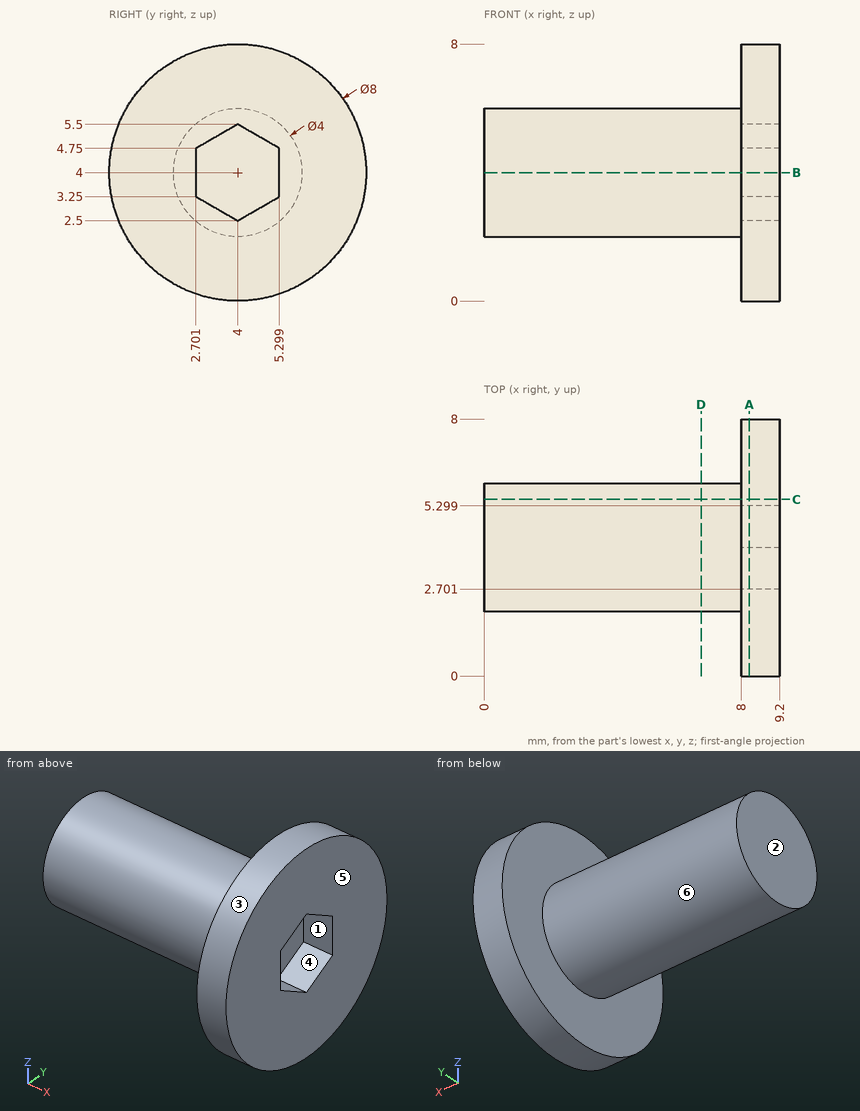
Could you check a few things on this drawing? It's one solid part, dimensions in mm from its lowest x, y, z. A direction names the side the tool comes from. Round coordinates to 2 decimals unless told otherwise and drop trailing zeros. Order: outer loops, then holes, each group sorted by start corner. A loop starts at its lowest first (then second) coordinate and runs counter-clockwise, first axis right, second up.
Q1. Imagine slicing it at C-C, the plane y = 5.5. List the corners of the cut face in (x, z) for me, then the cut area to 3 significant figures.
Geometry says:
outline: (0, 2.68) - (8, 2.68) - (8, 0.29) - (9.2, 0.29) - (9.2, 7.71) - (8, 7.71) - (8, 5.32) - (0, 5.32) - close
area: 30.1 mm2
Q2. Imagine slicing it at D-D, the plane x = 6.75. List the corners of the cut face in (y, z) for me, then the cut area to 3 significant figures.
Geometry says:
outline: circle Ø4 at (4, 4)
area: 12.6 mm2
Q3. I'm going to push flat-ended pins straight in: P1, Ø1.5, axis at y = 6.5, z = 2, coming from the -X side; P2, Ø1.3, axis at x = 8.5, z = 3.5, coming from the +Y side; P3, Ø2, axis at x = 3, y = 5, coming from the -Z side. Where does each tip first touch, or does it pass through?
Geometry says:
P1: stops at x = 8
P2: stops at y = 8
P3: stops at z = 2
Q4. Please list where these lines run through material, in increasing order: probe 1 along X at (y, z) = (4.5, 7.75); probe 2 along Y at (x, z) = (8.5, 5.25); probe 3 along Z at (x, y) = (2, 5.5).
Geometry says:
probe 1: x = 8 to 9.2
probe 2: y = 0.2 to 3.57, 4.43 to 7.8
probe 3: z = 2.68 to 5.32
Q5. Imagine slicing it at B-B, the plane z = 4. List the corners of the cut face in (x, y) for me.
Geometry says:
outline: (0, 2) - (8, 2) - (8, 0) - (9.2, 0) - (9.2, 2.7) - (8, 2.7) - (8, 5.3) - (9.2, 5.3) - (9.2, 8) - (8, 8) - (8, 6) - (0, 6) - close
Q6. Imagine slicing it at A-A, the plane x = 8.25. List the corners of the cut face in (y, z) for me, then the cut area to 3 significant figures.
Geometry says:
outline: circle Ø8 at (4, 4); hole (2.7, 3.25) - (4, 2.5) - (5.3, 3.25) - (5.3, 4.75) - (4, 5.5) - (2.7, 4.75) - close
area: 44.4 mm2
Q7. Which directions (+Z, -Z, +X, -X, +Y, -Y) give clear straight access to the entire face, cutting with the end or side of a thin tool? Please do the marked faces 4, 5 and 6.
Geometry says:
face 4: +X
face 5: +Z, -Z, +X, +Y, -Y
face 6: -X
Q8. Thinking about a two-plate mould opening in Z: for the marked faces 1, 2 and 3, which applies, released by +Z, released by -Z, zero draft, split by the parting line, or undercut?
Geometry says:
face 1: undercut
face 2: zero draft
face 3: split by the parting line
